Autodesk Inventor part; units mm, degrees
ref_plane "YZ Plane" through (0, 0, 0) normal (1, 0, 0) x (0, 1, 0)
ref_plane "XZ Plane" through (0, 0, 0) normal (0, 1, 0) x (-1, 0, 0)
ref_plane "XY Plane" through (0, 0, 0) normal (0, 0, 1) x (1, 0, 0)
sketch "Náčrt1" plane through (0, 0, 0) normal (0, 0, 1) x (1, 0, 0)
  line L0 (0, 0) -> (18.405, 0)
  line L1 (0, 20.165) -> (0, 40)
  line L2 (0, 40) -> (10, 40)
  line L3 (10, 40) -> (10, 37.25)
  line L4 (10, 37.25) -> (16, 37.25)
  line L5 (16, 37.25) -> (16, 20.165)
  line L6 (16, 20.165) -> (0, 20.165)
  dimension "d0" = 80
  dimension "d1" = 40.33
  dimension "d2" = 74.5
  dimension "d3" = 16
  dimension "d4" = 10
revolve "Rotace1" add sketch "Náčrt1" angle 360 about axis through (0, 0, 0) along (1, 0, 0)
fillet "Zaoblení1" radius 3 1 edges at (16, -20.165, 0)
fillet "Zaoblení2" radius 0.5 1 edges at (0, -20.165, 0)
chamfer "Zkosení1" distance 0.5 angle 45 2 edges at (0, -40, 0) (10, -40, 0)
equation "\"PoloměrOhybu\" = Tloušťka"
equation "\"ŠířkaVýštipu\" = Tloušťka"
equation "\"HloubkaVýštipu\" = 0.5 * Tloušťka"
equation "\"VelikostRohovéhoVýštipu\" = 4 * Tloušťka"
equation "\"MinimálníZbytek\" = 2 * Tloušťka"
equation "\"PřechodovýPoloměr\" = PoloměrOhybu"
equation "\"VelikostJacobihoPoloměru\" = Tloušťka"
equation "\"VelikostMezery\" = Tloušťka"
equation "\"Rozmer_B\" = 0"
equation "\"Rozmer_C\" = Tloušťka"
equation "\"Rozmer_D\" = d3"
properties part number "NA-45-h-Crown-217" material "19 436.4"
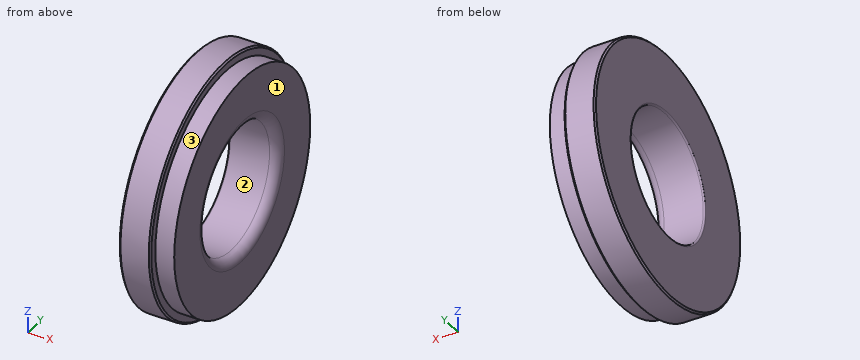
Design review of the part built by this model. Coordinates are the model's own, in mm. Face numbers are marked on the shaded views. Round coordinates to 2 decimals unless told otherwise and drop trailing zeros. Loops run counter-clockwise (first coordinate to the right, second up) from the corner with the lowest first, then second, coordinate; pieces in that order, holes last. Notation, with made-up numbers: (51, 58.5) - (58, 58.5) arc R26 cw to (58, 86.5) - close; hole circle Ø4 at (-32.75, -28). An arc over 180 degrees is marked (long way). One line per item, written item: value. Start each with the question number.
1) Insertion check: pin 1 Ø1.5 at (x, y) = (13.5, -9) entering from -Z; pin 2 Ø2 at (x, y) = (14, 24.5) entering from -Z; pin 3 Ø1 at (x, y) = (9, -28.5) entering from -Z. Each pin has a flat end and moves straight along its axis. Give the tip position at first contact, or say it passes through.
2) Consider section D-D on x = 6.25. Give the boundary of the cut face in (y, z) (3 decimals), then the cut area to 3 significant figures.
3) Consider section C-C on x = 12. Give the boundary of the cut face in (y, z) (3 decimals), then the cut area to 3 significant figures.
4) Draft analysis for pull direction Z (two halves, no side actions). For the marked faces 1, 2 and 3, state which applies: +Z half, -Z half, draft (parallel to the pull), parting line (faces both ways), or undercut.
5) To check wall thickness, follow L1, parallel to Z at x = 7.25, y = 0 (3 decimals); L2, parallel to Y at x = 11.5, z = 17; L3, parallel to X at y = -17, z = -33.5. State the ranges of each line that lie inside material, in increasing order. Write a range as from..to.
6) Consider section A-A on y = 0. Give the boundary of the cut face in (x, z) (3 decimals), then the cut area to 3 significant figures.
Reported:
1. pin 1: stops at z = -36.32
1. pin 2: stops at z = -28.9
1. pin 3: stops at z = -28.57
2. outline: circle Ø80 at (0, 0); hole circle Ø40.33 at (0, 0)
2. area: 3,750 mm^2
3. outline: circle Ø74.5 at (0, 0); hole circle Ø40.33 at (0, 0)
3. area: 3,080 mm^2
4. face 1: draft
4. face 2: undercut
4. face 3: parting line
5. L1: z = -40..-20.165, 20.165..40
5. L2: y = -33.14..-10.85, 10.85..33.14
5. L3: x = 0..10
6. outline: (0, -39.5) - (0.5, -40) - (9.5, -40) - (10, -39.5) - (10, -37.25) - (16, -37.25) - (16, -23.165) arc R3 ccw to (13, -20.165) - (0.5, -20.165) arc R0.5 ccw to (0, -20.665) - close; (0, 20.665) arc R0.5 ccw to (0.5, 20.165) - (13, 20.165) arc R3 ccw to (16, 23.165) - (16, 37.25) - (10, 37.25) - (10, 39.5) - (9.5, 40) - (0.5, 40) - (0, 39.5) - close
6. area: 597 mm^2
